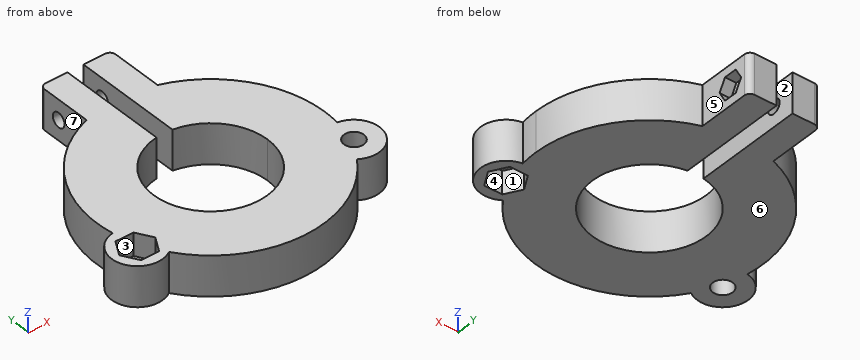
from build123d import *

# Parameters (mm, degrees)
F1_DEPTH  = 14
F3_DEPTH  = 25
F4_R      = 9
F5_DEPTH  = 14
F6_R      = 3.5
F7_DEPTH  = 25
F8_R      = 2.5
F9_DEPTH  = 25
F11_DEPTH = 4
F13_DEPTH = 8
F15_DEPTH = 8
F16_R     = 2


with BuildPart() as f1:
    # F0 (on Top) → F1 (new body)
    with BuildSketch(Plane.XY):
        with BuildLine():
            ThreePointArc((-12.5, 37.9967103839), (-23.4520787991, -32.403703492), (40, 0))
            ThreePointArc((40, 0), (32.403703492, 23.4520787991), (12.5, 37.9967103839))
            Line((12.5, 37.9967103839), (-12.5, 37.9967103839))
        make_face()
        with BuildLine():
            Line((-12.5, 37.9967103839), (12.5, 37.9967103839))
            ThreePointArc((12.5, 37.9967103839), (0, 40), (-12.5, 37.9967103839))
        make_face()
        with BuildLine():
            ThreePointArc((-12.5, 37.9967103839), (0, 40), (12.5, 37.9967103839))
            Line((12.5, 37.9967103839), (12.5, 57.9967103839))
            Line((12.5, 57.9967103839), (-12.5, 57.9967103839))
            Line((-12.5, 57.9967103839), (-12.5, 37.9967103839))
        make_face()
    extrude(amount=F1_DEPTH)

    # F2 (on face) → F3 (cut)
    with BuildSketch(Plane.XY.offset(14)):
        with BuildLine():
            ThreePointArc((-2.807373056, 19.8019861762), (-13.112065796, -15.102110136), (20, 0))
            ThreePointArc((20, 0), (15.102110136, 13.112065796), (2.807373056, 19.8019861762))
            Line((2.807373056, 19.8019861762), (-2.807373056, 19.8019861762))
        make_face()
        with BuildLine():
            Line((-2.807373056, 19.8019861762), (2.807373056, 19.8019861762))
            ThreePointArc((2.807373056, 19.8019861762), (0, 20), (-2.807373056, 19.8019861762))
        make_face()
        with BuildLine():
            ThreePointArc((-2.807373056, 19.8019861762), (0, 20), (2.807373056, 19.8019861762))
            Line((2.807373056, 19.8019861762), (2.807373056, 57.9967103839))
            Line((2.807373056, 57.9967103839), (-2.807373056, 57.9967103839))
            Line((-2.807373056, 57.9967103839), (-2.807373056, 19.8019861762))
        make_face()
    extrude(amount=-F3_DEPTH, mode=Mode.SUBTRACT)

    # F4 (on Top) → F5 (join)
    with BuildSketch(Plane.XY):
        with Locations((-38.1575680567, -15)):
            Circle(F4_R)
        with Locations((38.1575680567, -15)):
            Circle(F4_R)
    extrude(amount=F5_DEPTH)

    # F6 (on face) → F7 (cut)
    with BuildSketch(Plane.XY.offset(14)):
        with Locations((-38.1575680567, -15)):
            Circle(F6_R)
        with Locations((38.1575680567, -15)):
            Circle(F6_R)
    extrude(amount=-F7_DEPTH, mode=Mode.SUBTRACT)

    # F8 (on face) → F9 (cut)
    with BuildSketch(Plane(origin=(-12.5, 0, 0), x_dir=(0, -1, 0), z_dir=(-1, 0, 0))):
        with Locations((-49.9967103839, 7)):
            Circle(F8_R)
    extrude(amount=-F9_DEPTH, mode=Mode.SUBTRACT)

    # F10 (on face) → F11 (cut)
    with BuildSketch(Plane.YZ.offset(12.5)):
        Polygon((54.6155125374, 7), (52.3061114607, 11), (47.6873093072, 11), (45.3779082304, 7), (47.6873093072, 3), (52.3061114607, 3), align=None)
    extrude(amount=-F11_DEPTH, mode=Mode.SUBTRACT)

    # F12 (on face) → F13 (cut)
    with BuildSketch(Plane(origin=(0, 0, 0), x_dir=(1, 0, 0), z_dir=(0, 0, -1))):
        Polygon((41.3329945372, 20.5), (34.9821415761, 20.5), (31.8067150956, 15), (34.9821415761, 9.5), (41.3329945372, 9.5), (44.5084210178, 15), align=None)
    extrude(amount=-F13_DEPTH, mode=Mode.SUBTRACT)

    # F14 (on face) → F15 (cut)
    with BuildSketch(Plane.XY.offset(14)):
        Polygon((-31.8067150956, -15), (-34.9821415761, -9.5), (-41.3329945372, -9.5), (-44.5084210178, -15), (-41.3329945372, -20.5), (-34.9821415761, -20.5), align=None)
    extrude(amount=-F15_DEPTH, mode=Mode.SUBTRACT)

    # F16
    f16_edges = [f1.edges().sort_by_distance(p)[0] for p in [
        (12.5, 57.99671, 7),
        (-12.5, 57.99671, 7),
    ]]
    fillet(f16_edges, radius=F16_R)


solid = f1.part
Verification items for the finished model (mm, model axes). Face numbers are marked on the shaded views. A direction names the side the tool comes from. Give positions to 0.01 mm unless a question says otherwise; leave off trailing zeros. Write each loop counter-clockwise with the first axis right and the second up, starting at its lowest first coordinate (ties: lowest second). Pieces come first, ordered by that corner, then holes.
(1) Access from +Z, -Z, +X, -X, +Y, -Y to the whole of each face (thin tool, end or side, straight path). Record for the marked faces 1, 2 and 3.
(2) Mould release check, pull along X, two halves, no side actions. Record for the marked faces 4, 5, 6 and 7: +X half, -X half, draft (parallel to the pull), parting line (faces both ways), or undercut.
(3) Cross-section at C-C (z = 12.75). Enter the section's corners in (x, y).
(4) Cross-section at B-B (y = 5.5). Enter the section's corners in (x, z), plus the area to 3 significant figures.
(5) Cross-section at A-A (x = -5). Enter the section's corners in (y, z), plus the area to 3 significant figures.
(6) Gauge pin test, flat ends, axial feed: pin 1 (8 mm diameter, centred on x = -12.5, z = 9.5, fed in from +Y); pin 2 (5.5 mm diameter, centred on x = 38.16, y = -15, fed in from -Z); pin 3 (7 mm diameter, centred on y = 49, z = 4, fed in from +X); pin 4 (2.5 mm diameter, centred on y = 52, z = 7, fed in from +X). Record the tip position at first contact, or that the pin passes through.
(7) Material ranges on line 1 (Y direction, x = -4, z = 7.25); line 2 (Y direction, x = 3, z = 5); line 3 (X direction, y = 42, z = 2.75), recorded low to high.
Worked out:
1. face 1: -Z
1. face 2: +Z, -Z, +Y
1. face 3: +Z
2. face 4: undercut
2. face 5: +X half
2. face 6: draft
2. face 7: -X half
3. outline: (-39.53, -6.11) arc R9 ccw (long way) to (-33.11, -22.45) arc R40 ccw to (33.11, -22.45) arc R9 ccw (long way) to (39.53, -6.11) arc R40 ccw to (12.5, 38) - (12.5, 56) arc R2 ccw to (10.5, 58) - (2.81, 58) - (2.81, 19.8) arc R20 cw (long way) to (-2.81, 19.8) - (-2.81, 58) - (-10.5, 58) arc R2 ccw to (-12.5, 56) - (-12.5, 38) arc R40 ccw to start; hole (-44.51, -15) - (-41.33, -20.5) - (-34.98, -20.5) - (-31.81, -15) - (-34.98, -9.5) - (-41.33, -9.5) - close; hole circle Ø7 at (38.16, -15)
4. outline: (-39.62, 0) - (-19.23, 0) - (-19.23, 14) - (-39.62, 14) - close; (19.23, 0) - (39.62, 0) - (39.62, 14) - (19.23, 14) - close
4. area: 571 mm2
5. outline: (-39.69, 0) - (-19.36, 0) - (-19.36, 14) - (-39.69, 14) - close; (19.36, 0) - (58, 0) - (58, 14) - (19.36, 14) - close; hole circle Ø5 at (50, 7)
5. area: 806 mm2
6. pin 1: stops at y = 58
6. pin 2: passes through
6. pin 3: stops at x = 12.5
6. pin 4: stops at x = 8.5
7. line 1: y = -39.8 to -19.6, 19.6 to 47.51, 52.48 to 58
7. line 2: y = -39.89 to -19.77, 19.77 to 48.5, 51.5 to 58
7. line 3: x = -12.5 to -2.81, 2.81 to 12.5
